Study the drawing (mm; zero at the part's minimum x, y, z) and answer. Round coordinates to 2 decimals unless told otherwise and drop trailing zeros. Loops run counter-clockwise (first coordinate to the right, second up) from the corner with the lowest first, then second, coordinate; pieces in that order, holes last. Notation, with made-up numbers: (-15, -40) -> (15, -40) arc R20 cw to (15, -19) -> close; hole circle Ø11 at (82, 31.5). An arc over 180 degrees is marked (long way). Use one line per item in the form item = value.
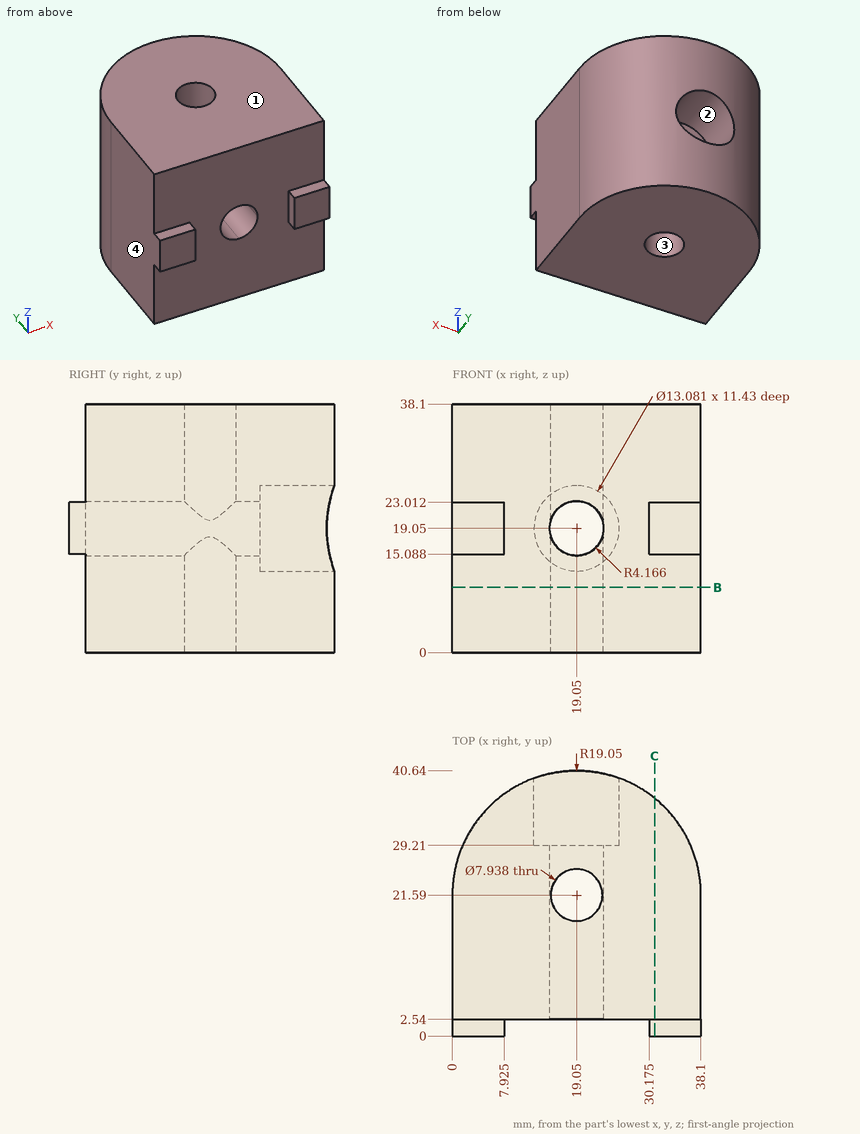
(1) Given P1, Ø17, axis at x = 19.05, z = 19.05, coming from the -Y side; P2, Ø3, axis at x = 33, y = 1, coming from the +Z side; P3, Ø4, axis at x = 23.5, z = 20.5, coming from the +Y side (1 decimal), each flat-ended and moving along its own axis, determine where each tip first touches the part or whether it passes through.
Completed:
P1 = 2.54
P2 = 23.01
P3 = 39.7
(2) Find section C-C, the plane x = 31. Write down the section's boundary in (y, z) (1 decimal).
Completed:
outline = (0, 15.1) -> (2.5, 15.1) -> (2.5, 0) -> (36.4, 0) -> (36.4, 38.1) -> (2.5, 38.1) -> (2.5, 23) -> (0, 23) -> close
(3) For a pull along X with two mould halves and no side action, classify the marked faces 1, 2, 3 and 4 as +X half, -X half, draft (parallel to the pull), parting line (faces both ways), or undercut.
Completed:
face_1 = draft
face_2 = undercut
face_3 = undercut
face_4 = -X half
(4) Consider L1, parallel to Y at x = 19.05, z = 12.25; L2, parallel to Z at x = 24, y = 36 (1 decimal); L3, parallel to X at y = 21, z = 29 (1 decimal). Determine where each line is inside the solid, lowest interval first.
Completed:
L1 = 2.54 to 17.62, 25.56 to 40.64
L2 = 0 to 14.8, 23.3 to 38.1
L3 = 0 to 15.1, 23 to 38.1
(5) Find section B-B, the plane z = 10. Write down the section's boundary in (x, y).
Completed:
outline = (0, 2.54) -> (38.1, 2.54) -> (38.1, 21.59) arc R19.05 ccw to (0, 21.59) -> close; hole circle Ø7.94 at (19.05, 21.59)
